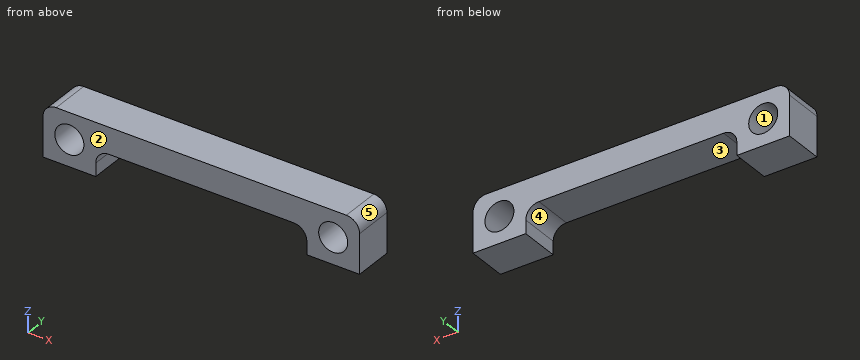
from build123d import *

# Parameters (mm, degrees)
F1_DEPTH = 38.1
F2_R     = 13.97
F3_DEPTH = 38.101


with BuildPart() as f1:
    # F0 (on Front) → F1 (new body)
    with BuildSketch(Plane.XZ):
        with BuildLine():
            Line((139.7, 25.4), (-139.7, 25.4))
            ThreePointArc((-139.7, 25.4), (-148.680256, 21.680256), (-152.4, 12.7))
            Line((-152.4, 12.7), (-152.4, -25.4))
            Line((-152.4, -25.4), (-101.6, -25.4))
            Line((-101.6, -25.4), (-101.6, -12.7))
            ThreePointArc((-101.6, -12.7), (-97.880256, -3.719744), (-88.9, 0))
            Line((-88.9, 0), (88.9, 0))
            ThreePointArc((88.9, 0), (97.880256, -3.719744), (101.6, -12.7))
            Line((101.6, -12.7), (101.6, -25.4))
            Line((101.6, -25.4), (152.4, -25.4))
            Line((152.4, -25.4), (152.4, 12.7))
            ThreePointArc((152.4, 12.7), (148.680256, 21.680256), (139.7, 25.4))
        make_face()
    extrude(amount=F1_DEPTH)

    # F2 (on face) → F3 (cut, through all)
    with BuildSketch(Plane.XZ.offset(38.1)):
        with Locations((-127, 0)):
            Circle(F2_R)
        with Locations((127, 0)):
            Circle(F2_R)
    extrude(amount=-F3_DEPTH, mode=Mode.SUBTRACT)


solid = f1.part
Design review of the part built by this model. Coordinates are the model's own, in mm. Face numbers are marked on the shaded views. A direction names the side the tool comes from. Coordinates: 2 decimals unless noted, no trailing zeros. Loops run counter-clockwise (first coordinate to the right, second up) from the corner with the lowest first, then second, coordinate; pieces in that order, holes last. Notation, with made-up numbers: M 46.25,30.5 L 74.25,30.5 A3 cw 74.25,34.5 Z; hole C 42.5,33 d5. An arc over 180 degrees is marked long. Use one line per item in the form item = value.
(1) Clearance check with flat-ended pins moving along their axes: P1, Ø17, axis at x = 127, z = 0, coming from the +Y side; P2, Ø4, axis at x = 26, y = -10, coming from the -Z side. State where each tip first meets the part, or that it passes through.
Return value:
P1 = through
P2 = 0
(2) Draft analysis for pull direction Z (two halves, no side actions). For the marked faces 1, 2 and 3, state which applies: pulls with the +Z half, pulls with the -Z half, needs draft (parallel to the pull), parting line crosses it, or undercut.
Return value:
face_1 = undercut
face_2 = needs draft
face_3 = pulls with the -Z half
(3) Consider section B-B (x = 127). Write out the cut boundary in (y, z).
Return value:
outline = M -38.1,-25.4 L 0,-25.4 L 0,-13.97 L -38.1,-13.97 Z; M -38.1,13.97 L 0,13.97 L 0,25.4 L -38.1,25.4 Z
(4) Consider section A-A (z = -16.5). Write out the cut boundary in (x, y), and give its area (3 significant figures).
Return value:
outline = M -152.4,-38.1 L -101.6,-38.1 L -101.6,0 L -152.4,0 Z; M 101.6,-38.1 L 152.4,-38.1 L 152.4,0 L 101.6,0 Z
area = 3,870 mm2
(5) For line 1 along X through (y, z) = (-9.5, -5); line 2 along Z through (x, y) = (127, -9); line 3 along X through (y, z) = (-7, 3), list the stretches that pass through material, from the lowest coordinate up. Write a range as from..to.
Return value:
line_1 = -152.4..-140.04, -113.96..-99, 99..113.96, 140.04..152.4
line_2 = -25.4..-13.97, 13.97..25.4
line_3 = -152.4..-140.64, -113.36..113.36, 140.64..152.4
(6) Consider section D-D (z = 6). Write out the cut boundary in (x, y).
Return value:
outline = M -152.4,-38.1 L -139.62,-38.1 L -139.62,0 L -152.4,0 Z; M -114.38,-38.1 L 114.38,-38.1 L 114.38,0 L -114.38,0 Z; M 139.62,-38.1 L 152.4,-38.1 L 152.4,0 L 139.62,0 Z
(7) Consider section C-C (y = -30.5). Write out the cut boundary in (x, z).
Return value:
outline = M -152.4,-25.4 L -101.6,-25.4 L -101.6,-12.7 A12.7 cw -88.9,0 L 88.9,0 A12.7 cw 101.6,-12.7 L 101.6,-25.4 L 152.4,-25.4 L 152.4,12.7 A12.7 ccw 139.7,25.4 L -139.7,25.4 A12.7 ccw -152.4,12.7 Z; hole C -127,0 d27.94; hole C 127,0 d27.94
(8) For the marked faces 4 and 5, list the 3-axis set-ups (+Z, -Z, +X, -X, +Y, -Y) from which the entire face can be reached by the end or side of a thin tool; tool diameter is ignored.
Return value:
face_4 = -Z, +Y, -Y
face_5 = +Z, +X, +Y, -Y
